Design review of the part built by this model. Coordinates are the model's own, in mm. Face numbers are marked on the shaded views. A direction names the side the tool comes from. Coordinates: 2 decimals unless noted, no trailing zeros. Write each loop counter-clockwise with the first axis right and the second up, starting at its lowest first coordinate (ties: lowest second). Pieces come first, ordered by that corner, then holes.
Q1. Machinability: for the marked faces 1 and 2, which of the approach directions +Z, -Z, +X, -X, +Y, -Y give a long, thin tool a straight path to every point of the face, cutting with its end or side? Answer none if there is none.
Q2. To check wall thickness, follow probe 1 along Y at (x, z) = (20.59, 1.65); probe 2 along Y at (x, z) = (-2.5, 3.25); probe 3 along X at (y, z) = (-0.25, 3.25). State the ranges of each line that lie inside material, in increasing order.
Q3. Add section A-A, the plane x = -5.85. Give the boundary of the cut face in (y, z), plus the area to 3 significant figures.
Q4. The part is to be moulded in two halves that separate along X. For the marked faces 3, 4 and 5, say which applies: +X half, -X half, draft (parallel to the pull), parting line (faces both ways), or undercut.
Q5. Clearance check with flat-ended pins moving along their axes: pin 1 Ø5 at (x, y) = (-16.5, -7.5) entering from +Z; pin 2 Ø1.8 at (x, y) = (-20.59, 8.89) entering from -Z; pin 3 Ø3.5 at (x, z) = (0, 10.925) entering from -Y. State where each tip first meets the part, or that it passes through.
Q6. Add section C-C, the plane z = 8. Give the boundary of the cut face in (x, y), plus the area to 3 significant figures.
Q7. Add section B-B, the plane x = 20.59. Give the boundary of the cut face in (y, z).
Q8. Add section D-D, the plane y = -10.5. Give the boundary of the cut face in (x, z).
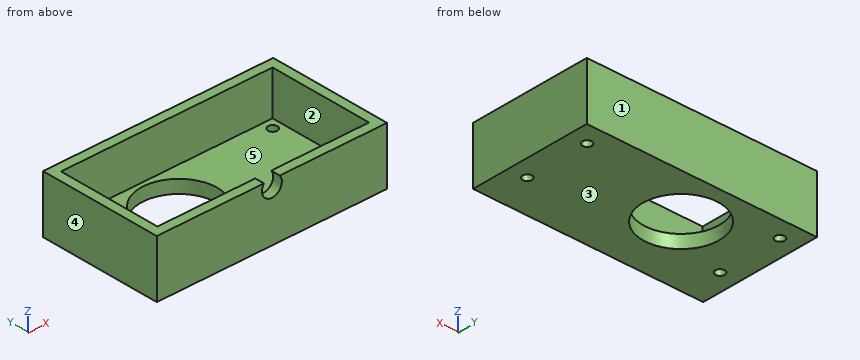
Autodesk Fusion 360 part; units mm, degrees
sketch "Boceto1" plane through (0, 0, 0) normal (0, 0, 1) x (1, 0, 0)
  line L0 (-22.6, -11.1) -> (22.6, -11.1)
  line L1 (22.6, -11.1) -> (22.6, 11.1)
  line L2 (22.6, 11.1) -> (-22.6, 11.1)
  line L3 (-22.6, 11.1) -> (-22.6, -11.1)
  line L4 (-22.6, -11.1) -> (22.6, 11.1) construction
  line L5 (22.6, -11.1) -> (-22.6, 11.1) construction
  circle A0 centre (-5.85, 2) radius 8.15
  circle A1 centre (-20.59, 8.89) radius 1
  line L6 (0, 11.1) -> (0, -11.1) construction
  line L7 (22.6, 13.1) -> (-22.6, 13.1)
  line L8 (-22.6, 13.1) -> (-22.6, 11.1)
  line L9 (-22.6, 11.1) -> (22.6, 11.1)
  line L10 (22.6, 11.1) -> (22.6, 13.1)
  line L11 (22.6, 13.1) -> (-22.6, 11.1) construction
  line L12 (-22.6, 13.1) -> (22.6, 11.1) construction
  line L13 (22.6, -13.1) -> (-22.6, -13.1)
  line L14 (-22.6, -13.1) -> (-22.6, -11.1)
  line L15 (-22.6, -11.1) -> (22.6, -11.1)
  line L16 (22.6, -11.1) -> (22.6, -13.1)
  line L17 (22.6, -13.1) -> (-22.6, -11.1) construction
  line L18 (-22.6, -13.1) -> (22.6, -11.1) construction
  line L19 (24.6, -13.1) -> (22.6, -13.1)
  line L20 (22.6, -13.1) -> (22.6, 13.1)
  line L21 (22.6, 13.1) -> (24.6, 13.1)
  line L22 (24.6, 13.1) -> (24.6, -13.1)
  line L23 (24.6, -13.1) -> (22.6, 13.1) construction
  line L24 (22.6, -13.1) -> (24.6, 13.1) construction
  line L25 (-22.6, -13.1) -> (-24.6, -13.1)
  line L26 (-24.6, -13.1) -> (-24.6, 13.1)
  line L27 (-24.6, 13.1) -> (-22.6, 13.1)
  line L28 (-22.6, 13.1) -> (-22.6, -13.1)
  line L29 (-22.6, -13.1) -> (-24.6, 13.1) construction
  line L30 (-24.6, -13.1) -> (-22.6, 13.1) construction
  circle A2 centre (-20.59, -4.89) radius 1
  circle A3 centre (20.59, 8.89) radius 1
  circle A4 centre (20.59, -4.89) radius 1
  point P0 (0, 12.1)
  point P1 (0, -12.1)
  point P2 (23.6, 0)
  point P3 (-23.6, 0)
  dimension "d5" = 22.2
  dimension "d6" = 45.2
  dimension "d7" = 16.3
  dimension "d10" = 2
  dimension "d11" = 2.01
  dimension "d12" = 2.21
  dimension "d13" = 45.2
  dimension "d14" = 2
  dimension "d15" = 45.2
  dimension "d16" = 2
  dimension "d17" = 2
  dimension "d18" = 26.2
  dimension "d19" = 2
  dimension "d20" = 26.2
  dimension "d26" = 16.75
  dimension "d27" = 9.1
  dimension "d28" = 2
  dimension "d29" = 2.01
  dimension "d30" = 6.21
extrude "Extruir1" add sketch "Boceto1" along normal blind 2.8 contours L0 L1 L2 L3 L9 L15 L20 L28
extrude "Extruir2" add sketch "Boceto1" along normal blind 12.2 contours L3 L8 L14 L25 L26 L27 L28 | L0 L13 L14 L15 L16 L20 L28 | L1 L10 L16 L19 L20 L21 L22 | L2 L7 L8 L9 L10 L20 L28
sketch "Boceto2" plane through (0, -13.1, 0) normal (0, -1, 0) x (1, 0, 0)
  line L0 (-24.6, 0) -> (24.6, 0)
  line L1 (24.6, 0) -> (24.6, 12.2)
  line L2 (24.6, 12.2) -> (-24.6, 12.2)
  line L3 (-24.6, 12.2) -> (-24.6, 0)
  arc A0 (-1.7, 12.2) -> (1.7, 12.2) centre (0, 10.925) ccw
  line L4 (-1.7, 12.2) -> (1.7, 12.2) construction
  line L5 (0, 12.2) -> (0, 8.8) construction
  dimension "d31" = 3.4
  dimension "d32" = 3.4
extrude "Extruir3" cut sketch "Boceto2" against normal blind 2 contours L2 A0
equation "grosor1 = 2.8 mm"
equation "grosor2 = 2 mm"
equation "grosor3 = 7.5 mm"
equation "tolerancia = 0.1 mm"
equation "d5 = 18 mm + tolerancia * 2 + margen_cable"
equation "d6 = 45 mm + tolerancia * 2"
equation "d7 = 16.2 mm + tolerancia"
equation "d10 = 1.9 mm + tolerancia"
equation "d11 = 1.91 mm + tolerancia"
equation "d12 = 2.11 mm + tolerancia"
equation "d13 = d6"
equation "d14 = grosor2"
equation "d15 = d6"
equation "d16 = grosor2"
equation "d17 = grosor2"
equation "d18 = d5 + grosor2 * 2"
equation "d19 = grosor2"
equation "d20 = d5 + grosor2 * 2"
equation "d21 = grosor1"
equation "d23 = 10.2 mm + grosor2"
equation "margen_cable = 4 mm"
equation "d28 = d10"
equation "d29 = d11"
equation "d30 = d12 + margen_cable"
equation "d33 = -grosor2"
Here are the results:
1. face 1: +Z, -Z, +X, -X, +Y
1. face 2: +Z
2. probe 1: y = -13.1 to -5.89, -3.89 to 7.89, 9.89 to 13.1
2. probe 2: y = -13.1 to -11.1, 11.1 to 13.1
2. probe 3: x = -24.6 to -22.6, 22.6 to 24.6
3. outline: (-13.1, 0) - (-6.15, 0) - (-6.15, 2.8) - (-11.1, 2.8) - (-11.1, 12.2) - (-13.1, 12.2) - close; (10.15, 0) - (13.1, 0) - (13.1, 12.2) - (11.1, 12.2) - (11.1, 2.8) - (10.15, 2.8) - close
3. area: 65.3 mm2
4. face 3: draft
4. face 4: -X half
4. face 5: undercut
5. pin 1: stops at z = 2.8
5. pin 2: passes through
5. pin 3: stops at y = 11.1
6. outline: (-24.6, -13.1) - (24.6, -13.1) - (24.6, 13.1) - (-24.6, 13.1) - close; hole (-22.6, -11.1) - (22.6, -11.1) - (22.6, 11.1) - (-22.6, 11.1) - close
6. area: 286 mm2
7. outline: (-13.1, 0) - (-5.89, 0) - (-5.89, 2.8) - (-11.1, 2.8) - (-11.1, 12.2) - (-13.1, 12.2) - close; (-3.89, 0) - (7.89, 0) - (7.89, 2.8) - (-3.89, 2.8) - close; (9.89, 0) - (13.1, 0) - (13.1, 12.2) - (11.1, 12.2) - (11.1, 2.8) - (9.89, 2.8) - close
8. outline: (-24.6, 0) - (24.6, 0) - (24.6, 12.2) - (22.6, 12.2) - (22.6, 2.8) - (-22.6, 2.8) - (-22.6, 12.2) - (-24.6, 12.2) - close
